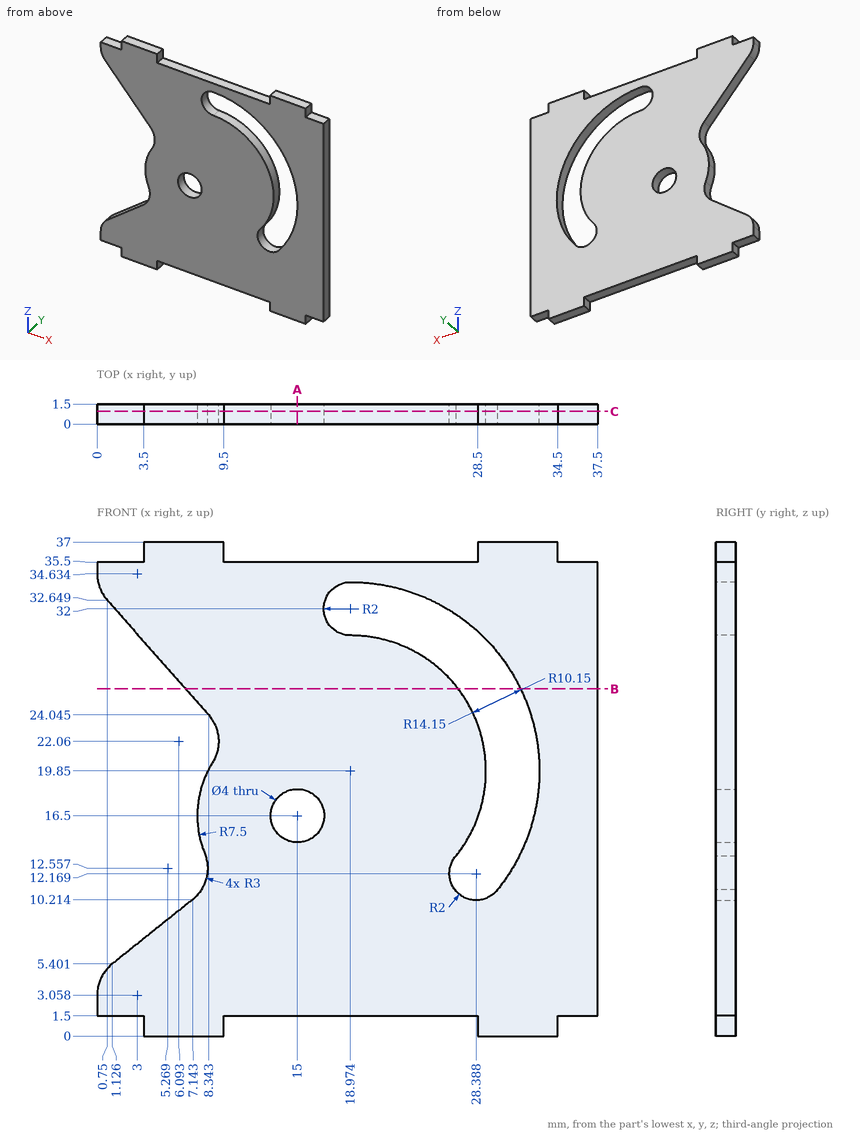
Source: three-view drawing plus pictorial views. Frame: mm from the lowest corner of the part. Give positions to 0.01 mm unless a question says otherwise; leave off trailing zeros. Order: outer loops, then holes, each group sorted by start corner. A loop starts at its lowest first (then second) coordinate and runs counter-clockwise, first axis right, second up. Notation, with made-up numbers: (42.5, 77) - (58.5, 77) arc R35 ccw to (58.5, 110) - close; hole circle Ø7 at (-10, 6). An arc over 180 degrees is marked (long way). Answer as a JSON object with one key per item and string values. Group by question number.
Q1. Cut plane B-B, the plane z = 26. Output: boundary loops of the cut face in (x, y).
Q2. First-contact query: pin 1 Ø0.8 at (y, z) = (0.5, 36) entering from -X; pin 2 Ø2.5 at (x, z) = (15, 16.5) entering from -Y; pin 3 Ø0.8 at (y, z) = (1, 36.5) entering from +X; pin 4 Ø0.8 at (x, y) = (36, 1) entering from -Z. Flat tips, straight axial feed; report the tip coordinate or a pass-through.
Q3. Cut plane C-C, the plane y = 0.95. Count the separate pieces of the cut face and the enclosed holes in it, then the cut area to 3 significant figures.
Q4. Cut plane A-A, the plane x = 15. Output: boundary loops of the cut face in (y, z).
Q5. Line query: probe 1 along Z at (x, y) = (15, 0.5); probe 2 along Z at (x, y) = (27.5, 0.5) (1 decimal); probe 3 along Z at (x, y) = (35, 1.1). Output: solid intervals per line, ascending.
Results:
{
 "1": {"outline": "(6.62, 0) - (27.05, 0) - (27.05, 1.5) - (6.62, 1.5) - close; (31.72, 0) - (37.5, 0) - (37.5, 1.5) - (31.72, 1.5) - close"},
 "2": {"pin 1": "x = 3.5", "pin 2": "through", "pin 3": "x = 34.5", "pin 4": "z = 1.5"},
 "3": {"separate pieces": "1", "enclosed holes": "2", "area": "1,000 mm^2"},
 "4": {"outline": "(0, 1.5) - (1.5, 1.5) - (1.5, 14.5) - (0, 14.5) - close; (0, 18.5) - (1.5, 18.5) - (1.5, 35.5) - (0, 35.5) - close"},
 "5": {"probe 1": "1.5 to 14.5, 18.5 to 35.5", "probe 2": "1.5 to 10.4, 14.3 to 25.4, 31.1 to 35.5", "probe 3": "1.5 to 35.5"}
}
